Could you check a few things on this model? Use its own coordinates, in mm. A direction names the side the tool comes from. Give positions to 0.01 mm unless a question says otherwise; leave off trailing zeros. Write each loop counter-clockwise with the first axis right and the second up, starting at its lowest first coordinate (ties: lowest second). Pieces come first, ordered by that corner, then holes. Notation, with made-up numbers: (-37.75, 54.25) -> (-32.75, 54.25) arc R29 cw to (-32.75, 85.25) -> close; hole circle Ø4 at (40, -6.75). An arc over 180 degrees is marked (long way). Write item = value, one per line. Start each with the question number.
```python
from build123d import *

# Parameters (mm, degrees)
BOSS_EXTRUDE1_DEPTH        = 13
F_2_7_2_7_DIAMETER_HOLE1_D = 2.7
SKETCH15_W                 = 18
SKETCH15_H                 = 2.5
CUT_EXTRUDE1_DEPTH         = 2.5


# Read off the part's stored shape, not the designer's step: CSK for M3 SFHCS1
with BuildPart() as part:
    # Sketch1 → Boss-Extrude1 (new body)
    with BuildSketch(Plane(origin=(0, 0, 0), x_dir=(1, 0, 0), z_dir=(0, 1, 0))):
        with BuildLine():
            Line((0, 9), (0, -9))
            Line((0, -9), (12, -9))
            ThreePointArc((12, -9), (7.32455532, 0), (12, 9))
            Line((12, 9), (0, 9))
        make_face()
    extrude(amount=BOSS_EXTRUDE1_DEPTH)

    # CSK for M3 SFHCS1 outline → CSK for M3 SFHCS1 (revolve, cut)
    with BuildSketch(Plane(origin=(0, 8, 0), x_dir=(0, 1, 0), z_dir=(0, 0, -1))):
        Polygon((1.7, 4.66), (1.7, 7.456784973), (0, 7.456784973), (0, 0), (3.36, 0), (3.36, 3), align=None)
    revolve(axis=Axis((0, 8, 0), (1, 0, 0)), mode=Mode.SUBTRACT)

    # Ø2.7 (2.7) Diameter Hole1 (through all)
    with Locations(Plane.ZY):
        with Locations((-6.75, 4), (6.75, 4)):
            Hole(F_2_7_2_7_DIAMETER_HOLE1_D / 2)

    # Sketch15 → Cut-Extrude1 (cut)
    with BuildSketch(Plane.ZY):
        with Locations((0, 11.75)):
            Rectangle(SKETCH15_W, SKETCH15_H)
    extrude(amount=-CUT_EXTRUDE1_DEPTH, mode=Mode.SUBTRACT)


solid = part.part
```
(1) Imagine slicing it at D-D (x = 3.5). Please give me the cut outline in (y, z), then the cut area to 3 significant figures.
(2) Imagine slicing it at A-A (y = 8). Please give me the cut outline in (x, z).
(3) Imagine slicing it at B-B (x = 2). Please give me the cut outline in (y, z).
(4) We'd pull the mould along Y, two halves only. Please class faces 1 (the cylindrical face through (6.08, 6.65, -1.03)), 2 (the flat face through (2.5, 12, 0)), 3 (the flat face through (6, 13, 0)): released by +Y, released by -Y, zero draft, split by the parting line, or undercut.
(5) I'm going to push flat-ended pins straight in: pin 1 (3 mm diameter, centred on y = 6.5, z = -7, fed in from -X); pin 2 (0.8 mm diameter, centred on x = 1.5, z = 7, fed in from +Y); pin 3 (5 mm diameter, centred on y = 10.5, z = 0.5, fed in from +X); pin 4 (1.5 mm diameter, centred on y = 11.5, z = -6.5, fed in from +X). Where does each tip first touch, or does it pass through?
(6) Imagine slicing it at C-C (z = 0). Please give me the cut outline in (x, y), then the cut area to 3 significant figures.
(7) If I drill on line 1 along Y through (x, z) = (6.5, -6.75); line 2 along Z through (x, y) = (3, 4); line 3 along Z through (x, y) = (5.95, 8), over which ranges is the centre line in solid material (lowest first)? Write a range as from..to.
(8) On a 3-axis mill with a long thin cutter (end or side, diameter ignored), from which of +Z, -Z, +X, -X, +Y, -Y can I reach the whole of each face in a straight line? I mean faces 4 (the cylindrical face through (1.521, 4.643, 0.148)), 5 (the flat face through (1, 10.5, 6)), 6 (the flat face through (0, 4, 0)). Say none if no direction works.
Answers below:
q1.outline = (0, -9) -> (13, -9) -> (13, 9) -> (0, 9) -> close; hole circle Ø2.7 at (4, -6.75); hole circle Ø2.7 at (4, 6.75); hole circle Ø5.72 at (8, 0)
q1.area = 197 mm^2
q2.outline = (0, -9) -> (12, -9) arc R11 cw to (7.46, -1.7) -> (4.66, -1.7) -> (3, -3.36) -> (0, -3.36) -> close; (0, 3.36) -> (3, 3.36) -> (4.66, 1.7) -> (7.46, 1.7) arc R11 cw to (12, 9) -> (0, 9) -> close
q3.outline = (0, -9) -> (10.5, -9) -> (10.5, -2.24) arc R3.36 cw (long way) to (10.5, 2.24) -> (10.5, 9) -> (0, 9) -> close; hole circle Ø2.7 at (4, -6.75); hole circle Ø2.7 at (4, 6.75)
q4.face_1 = undercut
q4.face_2 = zero draft
q4.face_3 = released by +Y
q5.pin_1 = 0
q5.pin_2 = 10.5
q5.pin_3 = 7.74
q5.pin_4 = 10.05
q6.outline = (0, 0) -> (7.32, 0) -> (7.32, 6.3) -> (4.66, 6.3) -> (3, 4.64) -> (0, 4.64) -> close; (2.5, 11.36) -> (3, 11.36) -> (4.66, 9.7) -> (7.32, 9.7) -> (7.32, 13) -> (2.5, 13) -> close
q6.area = 53.5 mm^2
q7.line_1 = 0..2.65, 5.35..13
q7.line_2 = -9..-8.1, -5.4..5.4, 8.1..9
q7.line_3 = -9..-1.7, 1.7..9
q8.face_4 = -X
q8.face_5 = +Z, -Z, -X, +Y
q8.face_6 = +Z, -Z, -X, +Y, -Y
